Design review of the part built by this model. Coordinates are the model's own, in mm. A direction names the side the tool comes from. Give positions to 0.01 mm unless a question says otherwise; leave off trailing zeros. Loops run counter-clockwise (first coordinate to the right, second up) from the corner with the lowest first, then second, coordinate; pieces in that order, holes last. Notation, with made-up numbers: (-24, 26) -> (9, 26) arc R36 ccw to (9, 63) -> close; hole circle Ø1 at (21, 15). An arc over 180 degrees is marked (long way). Answer in a Markdown table with one row per item. Add a question column.
(1) For faces 1 (the cylindrical face through (4.925, 8.964, 3.131)), 2 (the flat face through (1, 10.5, 3)), 3 (the flat face through (19, 10.5, 3)), 4 (the flat face through (5, 10.5, 3)), list the 3-axis set-ups (+Z, -Z, +X, -X, +Y, -Y) from which the entire face can be reached by the end or side of a thin tool; tool diameter is ignored.
(2) Consider section C-C on x = 5.25. Write out the cut boundary in (y, z).
(3) Consider section D-D on x = 10.25. Write out the cut boundary in (y, z).
(4) For line 1 (X direction, y = 11.25, z = 2) (1 decimal); line 2 (Y direction, x = 14.75, z = 3.25); line 3 (Y direction, x = 15.75, z = 5), list the stretches that pass through material, from the lowest coordinate up.
(5) Draft analysis for pull direction Y (two halves, no side actions). For faces 5 (the cylindrical face through (13.3, 8.4, 3.1)), 6 (the flat face through (9.462, -0.745, 3.219)), 7 (the flat face through (9.635, 12, 3)), state which applies: +Y half, -Y half, draft (parallel to the pull), parting line (faces both ways), or undercut.
(6) Consider section A-A on y = 12.75. Count the separate pieces of the cut face and the enclosed holes in it, then the cut area to 4 significant figures.
(7) For pin 1 (3 mm diameter, centred on y = 12.5, z = 2, fed in from +X); pin 2 (1.5 mm diameter, centred on x = 20.75, y = -1.53, fed in from +Z); pin 3 (1.8 mm diameter, centred on y = 12.5, z = 2, fed in from -X); pin 4 (3 mm diameter, centred on x = 3, z = 2, fed in from -Y), all flat-tipped, find the tip position at first contact; note any pin that passes through.
Autodesk Inventor part; units mm, degrees
ref_plane "YZ Plane" through (0, 0, 0) normal (1, 0, 0) x (0, 1, 0)
ref_plane "XZ Plane" through (0, 0, 0) normal (0, 1, 0) x (-1, 0, 0)
ref_plane "XY Plane" through (0, 0, 0) normal (0, 0, 1) x (1, 0, 0)
sketch "Sketch1" plane through (0, 0, 0) normal (0, 0, 1) x (1, 0, 0)
  line L0 (0, 0) -> (19.75, 0)
  line L1 (19.75, 0) -> (19.75, 10.5)
  line L2 (0, 10.5) -> (0, 0)
  line L3 (1.2485, 10.5) -> (1.2485, 14)
  line L4 (1.2485, 14) -> (1.7485, 14)
  line L5 (1.7485, 14) -> (1.7485, 10.5)
  line L6 (9.135, 10.5) -> (9.135, 14)
  line L7 (9.135, 14) -> (9.635, 14)
  line L8 (9.635, 14) -> (9.635, 10.5)
  line L9 (17.5504, 10.5) -> (17.5504, 14)
  line L10 (17.5504, 14) -> (17.0504, 14)
  line L11 (17.0504, 14) -> (17.0504, 10.5)
  line L12 (19.75, 10.5) -> (17.5504, 10.5)
  line L13 (17.0504, 10.5) -> (9.635, 10.5)
  line L14 (9.135, 10.5) -> (1.7485, 10.5)
  line L15 (1.2485, 10.5) -> (0, 10.5)
  line L16 (5.25, 7.5) -> (14.5, 7.5) construction
  circle A0 centre (5.25, 7.5) radius 1.5
  circle A1 centre (14.5, 7.5) radius 1.5
  dimension "d0" = 19.75
  dimension "d1" = 10.5
  dimension "d2" = 14
  dimension "d3" = 0.5
  dimension "d6" = 3
  dimension "d7" = 3
  dimension "d8" = 5.25
  dimension "d9" = 5.25
  dimension "d17" = 9.25
extrude "Extrusion1" add sketch "Sketch1" along normal blind 6.35
sketch "Sketch2" plane through (0, 0, 6.35) normal (0, 0, 1) x (1, 0, 0)
  line L0 (0, 0) -> (19.1921, -1.5105)
  line L1 (19.1921, -1.5105) -> (19.2157, -1.2105) construction
  line L2 (19.2157, -1.2105) -> (3.8355, 0)
  line L3 (0, 0) -> (19.75, 0)
  line L4 (0, 0) -> (3.8355, 0)
  arc A0 (19.1921, -1.5105) -> (22.3157, -1.4544) centre (20.7566, -1.6336) ccw
  line L5 (19.2157, -1.2105) -> (19.5157, -1.2341)
  line L6 (22.3157, -1.4544) -> (22.0157, -1.4308)
  arc A1 (19.5157, -1.2341) -> (22.0157, -1.4308) centre (20.75, -1.532) ccw
  line L7 (17.1531, -3.25) -> (26.6817, -3.25) construction
  line L8 (17.0504, 10.5) -> (9.635, 10.5)
  line L9 (19.75, 0) -> (19.75, 10.5)
  dimension "d10" = 0.3
  dimension "d11" = 13.75
  dimension "d12" = 4.5
  dimension "d13" = 2.5
  dimension "d14" = 1
extrude "Extrusion2" add sketch "Sketch2" against normal up to surface (6.35 mm away)
properties part number "Micro Endstop Triggered"
Values follow:
| question | item | result |
|---|---|---|
| 1 | face 1 | +Z, -Z |
| 1 | face 2 | +Z, -Z, -X, +Y |
| 1 | face 3 | +Z, -Z, +X, +Y |
| 1 | face 4 | +Z, -Z, +Y |
| 2 | outline | (-0.41, 0) -> (-0.11, 0) -> (-0.11, 6.35) -> (-0.41, 6.35) -> close; (0, 0) -> (6, 0) -> (6, 6.35) -> (0, 6.35) -> close; (9, 0) -> (10.5, 0) -> (10.5, 6.35) -> (9, 6.35) -> close |
| 3 | outline | (-0.81, 0) -> (-0.5, 0) -> (-0.5, 6.35) -> (-0.81, 6.35) -> close; (0, 0) -> (10.5, 0) -> (10.5, 6.35) -> (0, 6.35) -> close |
| 4 | line 1 | 1.2 to 1.7, 9.1 to 9.6, 17.1 to 17.6 |
| 4 | line 2 | -1.16 to -0.86, 0 to 6.02, 8.98 to 10.5 |
| 4 | line 3 | -1.24 to -0.94, 0 to 6.67, 8.33 to 10.5 |
| 5 | face 5 | undercut |
| 5 | face 6 | -Y half |
| 5 | face 7 | draft |
| 6 | separate pieces | 3 |
| 6 | enclosed holes | 0 |
| 6 | area | 9.525 mm2 |
| 7 | pin 1 | x = 17.55 |
| 7 | pin 2 | through |
| 7 | pin 3 | x = 1.25 |
| 7 | pin 4 | y = -0.35 |
